```python
from build123d import *

# Parameters (mm, degrees)
BOSS_EXTRUDE1_DEPTH = 343.25
SKETCH2_R           = 2.1
CUT_EXTRUDE1_DEPTH  = 5
SKETCH3_R           = 2.1
CUT_EXTRUDE2_DEPTH  = 5
SKETCH4_R           = 2.75
CUT_EXTRUDE3_DEPTH  = 5


with BuildPart() as part:
    # Sketch1 → Boss-Extrude1 (new body)
    with BuildSketch(Plane.XY):
        Polygon((0, 0), (50, 0), (50, 2), (2, 2), (2, 50), (0, 50), align=None)
    extrude(amount=BOSS_EXTRUDE1_DEPTH)

    # Sketch2 → Cut-Extrude1 (cut, symmetric)
    with BuildSketch(Plane(origin=(0, 0, 0), x_dir=(0, 0, -1), z_dir=(1, 0, 0))):
        with Locations((-185.75, 19.25)):
            Circle(SKETCH2_R)
        with Locations((-215, 19.25)):
            Circle(SKETCH2_R)
        with Locations((-290, 19.25)):
            Circle(SKETCH2_R)
        with Locations((-320.75, 19.25)):
            Circle(SKETCH2_R)
    extrude(amount=CUT_EXTRUDE1_DEPTH, both=True, mode=Mode.SUBTRACT)

    # Sketch3 → Cut-Extrude2 (cut, symmetric)
    with BuildSketch(Plane(origin=(0, 0, 0), x_dir=(0, 0, -1), z_dir=(1, 0, 0))):
        with Locations((-18, 12)):
            Circle(SKETCH3_R)
        with Locations((-128, 12)):
            Circle(SKETCH3_R)
    extrude(amount=CUT_EXTRUDE2_DEPTH, both=True, mode=Mode.SUBTRACT)

    # Sketch4 → Cut-Extrude3 (cut, symmetric)
    with BuildSketch(Plane(origin=(0, 0, 0), x_dir=(1, 0, 0), z_dir=(0, 1, 0))):
        with Locations(Location((25, -12.5, 0), (0, 0, 270))):
            Circle(SKETCH4_R)
        with Locations(Location((25, -37.5, 0), (0, 0, 270))):
            Circle(SKETCH4_R)
    extrude(amount=CUT_EXTRUDE3_DEPTH, both=True, mode=Mode.SUBTRACT)


solid = part.part
```
Model file for the job. Use its own axes, mm. A direction names the side the tool comes from. Round coordinates to 2 decimals unless told otherwise and drop trailing zeros. Order: outer loops, then holes, each group sorted by start corner. A loop starts at its lowest first (then second) coordinate and runs counter-clockwise, first axis right, second up. Notation, with made-up numbers: M -15,55 L -7,55 A23 ccw -7,65 Z; hole C 66,39 d3. An arc over 180 degrees is marked long. Use CSV: the item, a comma, the result in double quotes.
Item 1: Saw through at B-B (x = 17). List the corners of the cut face in (y, z), plus the area to 4 significant figures.
Worked answers:
outline,"M 0,0 L 2,0 L 2,343.25 L 0,343.25 Z"
area,"686.5 mm²"
Item 2: Saw through at A-A (z = 137). List the corners of the cut face in (x, y).
Worked answers:
outline,"M 0,0 L 50,0 L 50,2 L 2,2 L 2,50 L 0,50 Z"
Item 3: Probe probe 1 along Y at (x, z) = (1.3, 290); probe 2 along X at (y, z) = (1.45, 12.5); probe 3 along Y at (x, z) = (1, 128). List the from-to ranges inside material, lowest first.
Worked answers:
probe 1,"0 to 17.15, 21.35 to 50"
probe 2,"0 to 22.25, 27.75 to 50"
probe 3,"0 to 9.9, 14.1 to 50"
Item 4: Which spindle directions (+Z, -Z, +X, -X, +Y, -Y) get a long thin tool onto all of the face, cutting with end or side? Do faces 1 (the face through (25.121, 1.014, 34.753)), 2 (the face through (26, 2, 169)). Say none if no direction does.
Worked answers:
face 1,"+Y, -Y"
face 2,"+Z, -Z, +X, +Y"
Item 5: Pin check, flat tips, straight feed: pin 1 (2 mm diameter, centred on x = 18.5, z = 244.5, fed in from +Y); pin 2 (3.5 mm diameter, centred on y = 12, z = 18, fed in from -X); pin 3 (5 mm diameter, centred on y = 19.25, z = 215, fed in from +X). Stop position of each tip, or through.
Worked answers:
pin 1,"y = 2"
pin 2,"through"
pin 3,"x = 2"
Item 6: Pull direction X, two halves, no side cores. Call faces 3 (the face through (0, 25, 169)), 4 (the face through (2, 26, 169)), 5 (the face through (27.727, 0.986, 12.142)): released by +X, released by -X, zero draft, split by the parting line, or undercut.
Worked answers:
face 3,"released by -X"
face 4,"released by +X"
face 5,"undercut"
